```python
from build123d import *

# Parameters (mm, degrees)
F0_R     = 9.525
F1_DEPTH = 19.05
F2_DEPTH = 50.8
F3_DEPTH = 38.1


with BuildPart() as f1:
    # F0 (on Top) → F1 (new body)
    with BuildSketch(Plane.XY):
        with BuildLine():
            Line((-60.325, -16.4977839421), (-22.225, -38.4948291982))
            ThreePointArc((-22.225, -38.4948291982), (0, -44.45), (22.225, -38.4948291982))
            Line((22.225, -38.4948291982), (60.325, -16.4977839421))
            ThreePointArc((60.325, -16.4977839421), (69.85, 0), (60.325, 16.4977839421))
            Line((60.325, 16.4977839421), (22.225, 38.4948291982))
            ThreePointArc((22.225, 38.4948291982), (0, 44.45), (-22.225, 38.4948291982))
            Line((-22.225, 38.4948291982), (-60.325, 16.4977839421))
            ThreePointArc((-60.325, 16.4977839421), (-69.85, 0), (-60.325, -16.4977839421))
        make_face()
        with Locations((-50.8, 0)):
            Circle(F0_R, mode=Mode.SUBTRACT)
        with BuildLine():
            ThreePointArc((6.35, 34.3428758988), (24.6957043329, 24.6957043329), (34.3428758988, 6.35))
            ThreePointArc((34.3428758988, 6.35), (34.7791644937, 3.1883133656), (34.925, 0))
            ThreePointArc((34.925, 0), (34.7791644937, -3.1883133656), (34.3428758988, -6.35))
            ThreePointArc((34.3428758988, -6.35), (24.6957043329, -24.6957043329), (6.35, -34.3428758988))
            ThreePointArc((6.35, -34.3428758988), (0, -34.925), (-6.35, -34.3428758988))
            ThreePointArc((-6.35, -34.3428758988), (-24.6957043329, -24.6957043329), (-34.3428758988, -6.35))
            ThreePointArc((-34.3428758988, -6.35), (-34.925, 0), (-34.3428758988, 6.35))
            ThreePointArc((-34.3428758988, 6.35), (-24.6957043329, 24.6957043329), (-6.35, 34.3428758988))
            ThreePointArc((-6.35, 34.3428758988), (0, 34.925), (6.35, 34.3428758988))
        make_face(mode=Mode.SUBTRACT)
        with Locations((50.8, 0)):
            Circle(F0_R, mode=Mode.SUBTRACT)
    extrude(amount=F1_DEPTH)

    # F0 (on Top) → F2 (join)
    with BuildSketch(Plane.XY):
        with BuildLine():
            ThreePointArc((-24.5934442484, 6.35), (-17.9605122421, 17.9605122421), (-6.35, 24.5934442484))
            Line((-6.35, 24.5934442484), (-6.35, 34.3428758988))
            ThreePointArc((-6.35, 34.3428758988), (-24.6957043329, 24.6957043329), (-34.3428758988, 6.35))
            Line((-34.3428758988, 6.35), (-30.5676609278, 6.35))
            Line((-30.5676609278, 6.35), (-24.5934442484, 6.35))
        make_face()
        with BuildLine():
            Line((-6.35, -34.3428758988), (-6.35, -24.5934442484))
            ThreePointArc((-6.35, -24.5934442484), (-17.9605122421, -17.9605122421), (-24.5934442484, -6.35))
            Line((-24.5934442484, -6.35), (-34.3428758988, -6.35))
            ThreePointArc((-34.3428758988, -6.35), (-24.6957043329, -24.6957043329), (-6.35, -34.3428758988))
        make_face()
        with BuildLine():
            Line((25.4, -6.35), (24.5934442484, -6.35))
            ThreePointArc((24.5934442484, -6.35), (17.9605122421, -17.9605122421), (6.35, -24.5934442484))
            Line((6.35, -24.5934442484), (6.35, -29.9044754356))
            Line((6.35, -29.9044754356), (6.35, -34.3428758988))
            ThreePointArc((6.35, -34.3428758988), (24.6957043329, -24.6957043329), (34.3428758988, -6.35))
            Line((34.3428758988, -6.35), (25.4, -6.35))
        make_face()
        with BuildLine():
            ThreePointArc((6.35, 24.5934442484), (17.9605122421, 17.9605122421), (24.5934442484, 6.35))
            Line((24.5934442484, 6.35), (34.3428758988, 6.35))
            ThreePointArc((34.3428758988, 6.35), (24.6957043329, 24.6957043329), (6.35, 34.3428758988))
            Line((6.35, 34.3428758988), (6.35, 25.4))
            Line((6.35, 25.4), (6.35, 24.5934442484))
        make_face()
    extrude(amount=F2_DEPTH)

    # F0 (on Top) → F3 (join)
    with BuildSketch(Plane.XY):
        with BuildLine():
            ThreePointArc((24.5934442484, -6.35), (25.1975542852, -3.2005090291), (25.4, 0))
            ThreePointArc((25.4, 0), (25.1975542852, 3.2005090291), (24.5934442484, 6.35))
            ThreePointArc((24.5934442484, 6.35), (17.9605122421, 17.9605122421), (6.35, 24.5934442484))
            ThreePointArc((6.35, 24.5934442484), (0, 25.4), (-6.35, 24.5934442484))
            ThreePointArc((-6.35, 24.5934442484), (-17.9605122421, 17.9605122421), (-24.5934442484, 6.35))
            ThreePointArc((-24.5934442484, 6.35), (-25.4, 0), (-24.5934442484, -6.35))
            ThreePointArc((-24.5934442484, -6.35), (-17.9605122421, -17.9605122421), (-6.35, -24.5934442484))
            ThreePointArc((-6.35, -24.5934442484), (0, -25.4), (6.35, -24.5934442484))
            ThreePointArc((6.35, -24.5934442484), (17.9605122421, -17.9605122421), (24.5934442484, -6.35))
        make_face()
        with BuildLine():
            ThreePointArc((0, 12.7), (8.9802561211, 8.9802561211), (12.7, 0))
            ThreePointArc((12.7, 0), (8.9802561211, -8.9802561211), (0, -12.7))
            ThreePointArc((0, -12.7), (-8.9802561211, -8.9802561211), (-12.7, 0))
            ThreePointArc((-12.7, 0), (-8.9802561211, 8.9802561211), (0, 12.7))
        make_face(mode=Mode.SUBTRACT)
        with BuildLine():
            ThreePointArc((24.5934442484, 6.35), (25.1975542852, 3.2005090291), (25.4, 0))
            ThreePointArc((25.4, 0), (25.1975542852, -3.2005090291), (24.5934442484, -6.35))
            Line((24.5934442484, -6.35), (25.4, -6.35))
            Line((25.4, -6.35), (34.3428758988, -6.35))
            ThreePointArc((34.3428758988, -6.35), (34.7791644937, -3.1883133656), (34.925, 0))
            ThreePointArc((34.925, 0), (34.7791644937, 3.1883133656), (34.3428758988, 6.35))
            Line((34.3428758988, 6.35), (24.5934442484, 6.35))
        make_face()
        with BuildLine():
            ThreePointArc((-6.35, 24.5934442484), (0, 25.4), (6.35, 24.5934442484))
            Line((6.35, 24.5934442484), (6.35, 25.4))
            Line((6.35, 25.4), (6.35, 34.3428758988))
            ThreePointArc((6.35, 34.3428758988), (0, 34.925), (-6.35, 34.3428758988))
            Line((-6.35, 34.3428758988), (-6.35, 24.5934442484))
        make_face()
        with BuildLine():
            Line((6.35, -29.9044754356), (6.35, -24.5934442484))
            ThreePointArc((6.35, -24.5934442484), (0, -25.4), (-6.35, -24.5934442484))
            Line((-6.35, -24.5934442484), (-6.35, -34.3428758988))
            ThreePointArc((-6.35, -34.3428758988), (0, -34.925), (6.35, -34.3428758988))
            Line((6.35, -34.3428758988), (6.35, -29.9044754356))
        make_face()
        with BuildLine():
            ThreePointArc((-24.5934442484, -6.35), (-25.4, 0), (-24.5934442484, 6.35))
            Line((-24.5934442484, 6.35), (-30.5676609278, 6.35))
            Line((-30.5676609278, 6.35), (-34.3428758988, 6.35))
            ThreePointArc((-34.3428758988, 6.35), (-34.925, 0), (-34.3428758988, -6.35))
            Line((-34.3428758988, -6.35), (-24.5934442484, -6.35))
        make_face()
    extrude(amount=F3_DEPTH)


solid = f1.part
```
Verification items for the finished model (mm, model axes). A direction names the side the tool comes from. Give positions to 0.01 mm unless a question says otherwise; leave off trailing zeros. Order: outer loops, then holes, each group sorted by start corner. A loop starts at its lowest first (then second) coordinate and runs counter-clockwise, first axis right, second up. Notation, with made-up numbers: M 29.5,64 L 78.5,64 A34 ccw 78.5,96 Z; hole C 12,40 d1. An arc over 180 degrees is marked long. Answer in a Markdown table with one row per item. Add a question column.
Item 1: Section check A-A, the plane z = 47. Enter the section's corners in (x, y) (3 decimals).
Item 2: Gauge pin test, flat ends, axial feed: pin 1 (10 mm diameter, centred on y = -17.5, z = 26.5, fed in from +X); pin 2 (10.5 mm diameter, centred on y = -30, z = 44, fed in from +X); pin 3 (2 mm diameter, centred on x = 9, z = 36, fed in from -Y); pin 4 (22 mm diameter, centred on x = -50.8, y = 0, fed in from -Z). Record the tip position at first contact, or that the pin passes through.
Item 3: Mould release check, pull along X, two halves, no side actions. Record for faces 4 (the flat face through (41.542, 27.342, 9.392)), 5 (the cylindrical face through (59.6, -3.65, 9.39)), 6 (the flat face through (6.35, -29, 44)), 7 (the flat face through (20, 21, 50.8)): released by +X, released by -X, zero draft, split by the parting line, or undercut.
Item 4: Section check C-C, the plane z = 30.5. Enter the section's corners in (x, y) (3 decimals).
Item 5: Tool access check on faces 1 (the cylindrical face through (17.83, 18.09, 44.36)), 2 (the flat face through (6.35, 30, 44)), 3 (the flat face through (-30, 6.35, 44)). Record the directions out of +Z, -Z, +X, -X, +Y, -Y that give a thin tool (end or side, any length) a straight path to the whole face; none if there is none.
Item 6: Scan lines: probe 1 along Y at (x, z) = (-50.8, 13) (3 decimals); probe 2 along Z at (x, y) = (-30, 33); probe 3 along X at (y, z) = (-0.5, 32.5). Record each from-to range of solid material in increasing order. Write a range as from..to.
Item 7: Section check D-D, the plane z = 12.5. Enter the section's corners in (x, y) (3 decimals), and give its area (3 significant figures).
Item 8: Section check B-B, the plane x = 46. Enter the section's corners in (y, z), and give its area (3 significant figures).
Filled sheet:
| question | item | result |
|---|---|---|
| 1 | outline | M -34.343,-6.35 A34.925 ccw -6.35,-34.343 L -6.35,-24.593 A25.4 cw -24.593,-6.35 Z; M -34.343,6.35 L -24.593,6.35 A25.4 cw -6.35,24.593 L -6.35,34.343 A34.925 ccw Z; M 6.35,-34.343 A34.925 ccw 34.343,-6.35 L 24.593,-6.35 A25.4 cw 6.35,-24.593 Z; M 6.35,24.593 A25.4 cw 24.593,6.35 L 34.343,6.35 A34.925 ccw 6.35,34.343 Z |
| 2 | pin 1 | stops at x = 32.61 |
| 2 | pin 2 | stops at x = 24.64 |
| 2 | pin 3 | stops at y = -34 |
| 2 | pin 4 | stops at z = 0 |
| 3 | face 4 | released by +X |
| 3 | face 5 | undercut |
| 3 | face 6 | undercut |
| 3 | face 7 | zero draft |
| 4 | outline | C 0,0 d69.85; hole C 0,0 d25.4 |
| 5 | face 1 | +Z |
| 5 | face 2 | +Z, +Y, -Y |
| 5 | face 3 | +Z, +X, -X |
| 6 | probe 1 | y = -21.997..-9.525, 9.525..21.997 |
| 6 | probe 2 | z = 0..19.05 |
| 6 | probe 3 | x = -34.92..-12.69, 12.69..34.92 |
| 7 | outline | M -60.325,-16.498 L -22.225,-38.495 A44.45 ccw 22.225,-38.495 L 60.325,-16.498 A19.05 ccw 60.325,16.498 L 22.225,38.495 A44.45 ccw -22.225,38.495 L -60.325,16.498 A19.05 ccw Z; hole C -50.8,0 d19.05; hole C 0,0 d25.4; hole C 50.8,0 d19.05 |
| 7 | area | 7,340 mm^2 |
| 8 | outline | M -24.77,0 L -8.23,0 L -8.23,19.05 L -24.77,19.05 Z; M 8.23,0 L 24.77,0 L 24.77,19.05 L 8.23,19.05 Z |
| 8 | area | 630 mm^2 |
